The listing builds one solid part. Answer for the finished solid, in the listing's coordinates (mm). Face numbers are marked on the shaded views. A direction names the side the tool comes from. Give positions to 0.01 mm unless a question says otherwise; leave off trailing zeros. Write each loop counter-clockwise with the first axis right and the second up, starting at its lowest first coordinate (ties: lowest second). Pieces come first, ordered by that corner, then holes. Notation, with made-up numbers: (59, 86) - (70, 86) arc R25 cw to (70, 102) - close; hole circle Ø2 at (6, 48). An arc over 180 degrees is marked (long way). Use a Markdown table: item, result. Add a question column.
Autodesk Inventor part; units mm, degrees
ref_plane "YZ Plane" through (0, 0, 0) normal (1, 0, 0) x (0, 1, 0)
ref_plane "XZ Plane" through (0, 0, 0) normal (0, 1, 0) x (-1, 0, 0)
ref_plane "XY Plane" through (0, 0, 0) normal (0, 0, 1) x (1, 0, 0)
sketch "Sketch1" plane through (0, 0, 0) normal (0, 1, 0) x (-1, 0, 0)
  circle A0 centre (0, 0) radius 8
  dimension "d0" = 16
extrude "Extrusion1" add sketch "Sketch1" along normal blind 150
sketch "Sketch2" plane through (0, 150, 0) normal (0, 1, 0) x (1, 0, 0)
  circle A0 centre (0, 0) radius 8
  circle A1 centre (0, 0) radius 5
  dimension "d3" = 10
extrude "Extrusion2" add sketch "Sketch2" along normal blind 17 contours A1
sketch "Sketch3" plane through (0, 167, 0) normal (0, 1, 0) x (1, 0, 0)
  circle A0 centre (0, 0) radius 5
  circle A1 centre (0, 0) radius 2
  dimension "d6" = 4
extrude "Extrusion3" add sketch "Sketch3" along normal blind 7 contours A1
fillet "Fillet1" radius 3 1 edges at (8, 150, 0)
fillet "Fillet2" radius 3 1 edges at (-5, 167, 0)
fillet "Fillet3" radius 2 1 edges at (-2, 174, 0)
properties part number "pen_pentel_knockle"
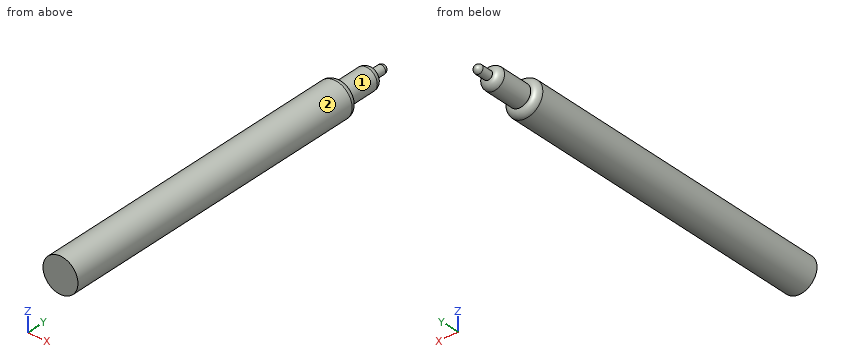
1. Consider L1, parallel to Z at x = 0.25, y = 10; L2, parallel to Y at x = -3.5, z = 4; L3, parallel to X at y = 118.5, z = -1.75. Determine where each line is inside the solid, lowest interval first. Write a range as [from, to].
2. The part is cut by section A-A (y = 121). Give the vertices of the cut face in (x, z).
3. Which of the six approach directions +Z, -Z, +X, -X, +Y, -Y give full straight-line access (tool end or side, diameter ignored) to the marked faces 1 and 2?
4. Given P1, Ø1, axis at x = 3.5, y = 126.5, coming from the +Z side; P2, Ø5, axis at y = 117.5, z = -5.5, coming from the +X side; P3, Ø5, axis at y = 108, z = 5, coming from the -X side, each flat-ended and moving along its own axis, determine where each tip first touches the part or whether it passes through.
Check values:
| question | item | result |
|---|---|---|
| 1 | L1 | z = [-8, 8] |
| 1 | L2 | y = [0, 149.98] |
| 1 | L3 | x = [-7.81, 7.81] |
| 2 | outline | circle Ø16 at (0, 0) |
| 3 | face 1 | +Y |
| 3 | face 2 | +Y, -Y |
| 4 | P1 | stops at z = 7.42 |
| 4 | P2 | stops at x = 7.42 |
| 4 | P3 | stops at x = -7.6 |
